For this review, take the finished solid that the model builds, in its own axes (mm). A direction names the side the tool comes from. Round coordinates to 2 decimals unless told otherwise and drop trailing zeros. Write each loop counter-clockwise with the first axis right and the second up, starting at its lowest first coordinate (ties: lowest second). Pieces come first, ordered by that corner, then holes. Notation, with made-up numbers: (-36.5, -24) -> (-13.5, -24) arc R22 cw to (-13.5, -4) -> close; hole circle Ø1 at (56.5, -25.75). An arc over 180 degrees is marked (long way). Answer as CSV lines item,"result". Start each with the question number.
Item 1: For pin 1 Ø1 at (y, z) = (0.5, 21) entering from +X (3 decimals); pin 2 Ø1.6 at (x, y) = (21.5, 1) entering from +Z (3 decimals), all flat-tipped, find the tip position at first contact; note any pin that passes through.
Item 2: Wall thickness on probe 1 along Z at (x, y) = (48.5, 3) (3 decimals); probe 2 along X at (y, z) = (0.25, 67.5) (3 decimals): over which ranges is each line inside the solid? List them lowest first. Write a range as from..to.
Item 3: Take a section at B-B on y = 1.45. Count the separate pieces of the cut face and the enclosed holes in it, then the cut area to 3 significant figures.
Item 4: Machinability: for faces 1 (the flat face through (2, 2, 23)), 2 (the flat face through (86, 2, 71)), 3 (the flat face through (24, 2, 21)), which of the approach directions +Z, -Z, +X, -X, +Y, -Y give a long, thin tool a straight path to every point of the face, cutting with its end or side? Answer none if there is none.
Item 5: Take a section at A-A on x = 69. Give the boundary of the cut face in (y, z) (3 decimals).
Item 6: Mouldability with a two-part tool opening along X and no side actions: class faces 4 (the flat face through (20, 2, 102.35)), 5 (the flat face through (0, 2, 55)), 6 (the flat face through (60, 2, 110)) as +X half, -X half, draft (parallel to the pull), parting line (faces both ways), or undercut.
```python
from build123d import *

# Parameters (mm, degrees)
SKETCH1_W           = 88
SKETCH1_H           = 110
BOSS_EXTRUDE1_DEPTH = 3.175
CUT_EXTRUDE1_REACH  = 5.175
SKETCH2_W           = 8
SKETCH2_H           = 3.175
SKETCH2_W_2         = 3.175
SKETCH2_H_2         = 8
CUT_EXTRUDE2_REACH  = 5.175
SKETCH3_W           = 8
SKETCH3_H           = 3.175
CUT_EXTRUDE3_REACH  = 5.175
SKETCH4_W           = 8
SKETCH4_H           = 3.175


with BuildPart() as part:
    # Sketch1 → Boss-Extrude1 (new body)
    with BuildSketch(Plane(origin=(0, 0, 0), x_dir=(1, 0, 0), z_dir=(0, 1, 0))):
        with Locations((44, -55)):
            Rectangle(SKETCH1_W, SKETCH1_H)
    extrude(amount=BOSS_EXTRUDE1_DEPTH)

    # Sketch2 → Cut-Extrude1 (cut, up to next)
    with BuildSketch(Plane(origin=(0, 3.175, 0), x_dir=(1, 0, 0), z_dir=(0, 1, 0)), mode=Mode.PRIVATE) as cut_extrude1_sk1:
        with Locations((68, -1.5875)):
            Rectangle(SKETCH2_W, SKETCH2_H)
    cut_extrude1_tool1 = extrude(cut_extrude1_sk1.sketch, amount=-CUT_EXTRUDE1_REACH, mode=Mode.PRIVATE) & part.part
    add(cut_extrude1_tool1.solids().sort_by_distance((68, 3.175, 1.5875))[0], mode=Mode.SUBTRACT)
    # Sketch2 → Cut-Extrude1 (cut, up to next)
    with BuildSketch(Plane(origin=(0, 3.175, 0), x_dir=(1, 0, 0), z_dir=(0, 1, 0)), mode=Mode.PRIVATE) as cut_extrude1_sk2:
        with Locations((52, -1.5875)):
            Rectangle(SKETCH2_W, SKETCH2_H)
    cut_extrude1_tool2 = extrude(cut_extrude1_sk2.sketch, amount=-CUT_EXTRUDE1_REACH, mode=Mode.PRIVATE) & part.part
    add(cut_extrude1_tool2.solids().sort_by_distance((52, 3.175, 1.5875))[0], mode=Mode.SUBTRACT)
    # Sketch2 → Cut-Extrude1 (cut, up to next)
    with BuildSketch(Plane(origin=(0, 3.175, 0), x_dir=(1, 0, 0), z_dir=(0, 1, 0)), mode=Mode.PRIVATE) as cut_extrude1_sk3:
        with Locations((20, -1.5875)):
            Rectangle(SKETCH2_W, SKETCH2_H)
    cut_extrude1_tool3 = extrude(cut_extrude1_sk3.sketch, amount=-CUT_EXTRUDE1_REACH, mode=Mode.PRIVATE) & part.part
    add(cut_extrude1_tool3.solids().sort_by_distance((20, 3.175, 1.5875))[0], mode=Mode.SUBTRACT)
    # Sketch2 → Cut-Extrude1 (cut, up to next)
    with BuildSketch(Plane(origin=(0, 3.175, 0), x_dir=(1, 0, 0), z_dir=(0, 1, 0)), mode=Mode.PRIVATE) as cut_extrude1_sk4:
        with Locations((36, -1.5875)):
            Rectangle(SKETCH2_W, SKETCH2_H)
    cut_extrude1_tool4 = extrude(cut_extrude1_sk4.sketch, amount=-CUT_EXTRUDE1_REACH, mode=Mode.PRIVATE) & part.part
    add(cut_extrude1_tool4.solids().sort_by_distance((36, 3.175, 1.5875))[0], mode=Mode.SUBTRACT)
    # Sketch2 → Cut-Extrude1 (cut, up to next)
    with BuildSketch(Plane(origin=(0, 3.175, 0), x_dir=(1, 0, 0), z_dir=(0, 1, 0)), mode=Mode.PRIVATE) as cut_extrude1_sk5:
        with Locations((1.5875, -19)):
            Rectangle(SKETCH2_W_2, SKETCH2_H_2)
    cut_extrude1_tool5 = extrude(cut_extrude1_sk5.sketch, amount=-CUT_EXTRUDE1_REACH, mode=Mode.PRIVATE) & part.part
    add(cut_extrude1_tool5.solids().sort_by_distance((1.5875, 3.175, 19))[0], mode=Mode.SUBTRACT)
    # Sketch2 → Cut-Extrude1 (cut, up to next)
    with BuildSketch(Plane(origin=(0, 3.175, 0), x_dir=(1, 0, 0), z_dir=(0, 1, 0)), mode=Mode.PRIVATE) as cut_extrude1_sk6:
        with Locations((1.5875, -43)):
            Rectangle(SKETCH2_W_2, SKETCH2_H_2)
    cut_extrude1_tool6 = extrude(cut_extrude1_sk6.sketch, amount=-CUT_EXTRUDE1_REACH, mode=Mode.PRIVATE) & part.part
    add(cut_extrude1_tool6.solids().sort_by_distance((1.5875, 3.175, 43))[0], mode=Mode.SUBTRACT)
    # Sketch2 → Cut-Extrude1 (cut, up to next)
    with BuildSketch(Plane(origin=(0, 3.175, 0), x_dir=(1, 0, 0), z_dir=(0, 1, 0)), mode=Mode.PRIVATE) as cut_extrude1_sk7:
        with Locations((1.5875, -91)):
            Rectangle(SKETCH2_W_2, SKETCH2_H_2)
    cut_extrude1_tool7 = extrude(cut_extrude1_sk7.sketch, amount=-CUT_EXTRUDE1_REACH, mode=Mode.PRIVATE) & part.part
    add(cut_extrude1_tool7.solids().sort_by_distance((1.5875, 3.175, 91))[0], mode=Mode.SUBTRACT)
    # Sketch2 → Cut-Extrude1 (cut, up to next)
    with BuildSketch(Plane(origin=(0, 3.175, 0), x_dir=(1, 0, 0), z_dir=(0, 1, 0)), mode=Mode.PRIVATE) as cut_extrude1_sk8:
        with Locations((1.5875, -67)):
            Rectangle(SKETCH2_W_2, SKETCH2_H_2)
    cut_extrude1_tool8 = extrude(cut_extrude1_sk8.sketch, amount=-CUT_EXTRUDE1_REACH, mode=Mode.PRIVATE) & part.part
    add(cut_extrude1_tool8.solids().sort_by_distance((1.5875, 3.175, 67))[0], mode=Mode.SUBTRACT)
    # Sketch2 → Cut-Extrude1 (cut, up to next)
    with BuildSketch(Plane(origin=(0, 3.175, 0), x_dir=(1, 0, 0), z_dir=(0, 1, 0)), mode=Mode.PRIVATE) as cut_extrude1_sk9:
        with Locations((20, -108.4125)):
            Rectangle(SKETCH2_W, SKETCH2_H)
    cut_extrude1_tool9 = extrude(cut_extrude1_sk9.sketch, amount=-CUT_EXTRUDE1_REACH, mode=Mode.PRIVATE) & part.part
    add(cut_extrude1_tool9.solids().sort_by_distance((20, 3.175, 108.4125))[0], mode=Mode.SUBTRACT)
    # Sketch2 → Cut-Extrude1 (cut, up to next)
    with BuildSketch(Plane(origin=(0, 3.175, 0), x_dir=(1, 0, 0), z_dir=(0, 1, 0)), mode=Mode.PRIVATE) as cut_extrude1_sk10:
        with Locations((36, -108.4125)):
            Rectangle(SKETCH2_W, SKETCH2_H)
    cut_extrude1_tool10 = extrude(cut_extrude1_sk10.sketch, amount=-CUT_EXTRUDE1_REACH, mode=Mode.PRIVATE) & part.part
    add(cut_extrude1_tool10.solids().sort_by_distance((36, 3.175, 108.4125))[0], mode=Mode.SUBTRACT)
    # Sketch2 → Cut-Extrude1 (cut, up to next)
    with BuildSketch(Plane(origin=(0, 3.175, 0), x_dir=(1, 0, 0), z_dir=(0, 1, 0)), mode=Mode.PRIVATE) as cut_extrude1_sk11:
        with Locations((68, -108.4125)):
            Rectangle(SKETCH2_W, SKETCH2_H)
    cut_extrude1_tool11 = extrude(cut_extrude1_sk11.sketch, amount=-CUT_EXTRUDE1_REACH, mode=Mode.PRIVATE) & part.part
    add(cut_extrude1_tool11.solids().sort_by_distance((68, 3.175, 108.4125))[0], mode=Mode.SUBTRACT)
    # Sketch2 → Cut-Extrude1 (cut, up to next)
    with BuildSketch(Plane(origin=(0, 3.175, 0), x_dir=(1, 0, 0), z_dir=(0, 1, 0)), mode=Mode.PRIVATE) as cut_extrude1_sk12:
        with Locations((52, -108.4125)):
            Rectangle(SKETCH2_W, SKETCH2_H)
    cut_extrude1_tool12 = extrude(cut_extrude1_sk12.sketch, amount=-CUT_EXTRUDE1_REACH, mode=Mode.PRIVATE) & part.part
    add(cut_extrude1_tool12.solids().sort_by_distance((52, 3.175, 108.4125))[0], mode=Mode.SUBTRACT)
    # Sketch2 → Cut-Extrude1 (cut, up to next)
    with BuildSketch(Plane(origin=(0, 3.175, 0), x_dir=(1, 0, 0), z_dir=(0, 1, 0)), mode=Mode.PRIVATE) as cut_extrude1_sk13:
        with Locations((86.4125, -91)):
            Rectangle(SKETCH2_W_2, SKETCH2_H_2)
    cut_extrude1_tool13 = extrude(cut_extrude1_sk13.sketch, amount=-CUT_EXTRUDE1_REACH, mode=Mode.PRIVATE) & part.part
    add(cut_extrude1_tool13.solids().sort_by_distance((86.4125, 3.175, 91))[0], mode=Mode.SUBTRACT)
    # Sketch2 → Cut-Extrude1 (cut, up to next)
    with BuildSketch(Plane(origin=(0, 3.175, 0), x_dir=(1, 0, 0), z_dir=(0, 1, 0)), mode=Mode.PRIVATE) as cut_extrude1_sk14:
        with Locations((86.4125, -67)):
            Rectangle(SKETCH2_W_2, SKETCH2_H_2)
    cut_extrude1_tool14 = extrude(cut_extrude1_sk14.sketch, amount=-CUT_EXTRUDE1_REACH, mode=Mode.PRIVATE) & part.part
    add(cut_extrude1_tool14.solids().sort_by_distance((86.4125, 3.175, 67))[0], mode=Mode.SUBTRACT)
    # Sketch2 → Cut-Extrude1 (cut, up to next)
    with BuildSketch(Plane(origin=(0, 3.175, 0), x_dir=(1, 0, 0), z_dir=(0, 1, 0)), mode=Mode.PRIVATE) as cut_extrude1_sk15:
        with Locations((86.4125, -19)):
            Rectangle(SKETCH2_W_2, SKETCH2_H_2)
    cut_extrude1_tool15 = extrude(cut_extrude1_sk15.sketch, amount=-CUT_EXTRUDE1_REACH, mode=Mode.PRIVATE) & part.part
    add(cut_extrude1_tool15.solids().sort_by_distance((86.4125, 3.175, 19))[0], mode=Mode.SUBTRACT)
    # Sketch2 → Cut-Extrude1 (cut, up to next)
    with BuildSketch(Plane(origin=(0, 3.175, 0), x_dir=(1, 0, 0), z_dir=(0, 1, 0)), mode=Mode.PRIVATE) as cut_extrude1_sk16:
        with Locations((86.4125, -43)):
            Rectangle(SKETCH2_W_2, SKETCH2_H_2)
    cut_extrude1_tool16 = extrude(cut_extrude1_sk16.sketch, amount=-CUT_EXTRUDE1_REACH, mode=Mode.PRIVATE) & part.part
    add(cut_extrude1_tool16.solids().sort_by_distance((86.4125, 3.175, 43))[0], mode=Mode.SUBTRACT)

    # Sketch3 → Cut-Extrude2 (cut, up to next)
    with BuildSketch(Plane(origin=(0, 3.175, 0), x_dir=(1, 0, 0), z_dir=(0, 1, 0)), mode=Mode.PRIVATE) as cut_extrude2_sk1:
        with Locations((68, -20.7625)):
            Rectangle(SKETCH3_W, SKETCH3_H)
    cut_extrude2_tool1 = extrude(cut_extrude2_sk1.sketch, amount=-CUT_EXTRUDE2_REACH, mode=Mode.PRIVATE) & part.part
    add(cut_extrude2_tool1.solids().sort_by_distance((68, 3.175, 20.7625))[0], mode=Mode.SUBTRACT)
    # Sketch3 → Cut-Extrude2 (cut, up to next)
    with BuildSketch(Plane(origin=(0, 3.175, 0), x_dir=(1, 0, 0), z_dir=(0, 1, 0)), mode=Mode.PRIVATE) as cut_extrude2_sk2:
        with Locations((52, -20.7625)):
            Rectangle(SKETCH3_W, SKETCH3_H)
    cut_extrude2_tool2 = extrude(cut_extrude2_sk2.sketch, amount=-CUT_EXTRUDE2_REACH, mode=Mode.PRIVATE) & part.part
    add(cut_extrude2_tool2.solids().sort_by_distance((52, 3.175, 20.7625))[0], mode=Mode.SUBTRACT)
    # Sketch3 → Cut-Extrude2 (cut, up to next)
    with BuildSketch(Plane(origin=(0, 3.175, 0), x_dir=(1, 0, 0), z_dir=(0, 1, 0)), mode=Mode.PRIVATE) as cut_extrude2_sk3:
        with Locations((20, -20.7625)):
            Rectangle(SKETCH3_W, SKETCH3_H)
    cut_extrude2_tool3 = extrude(cut_extrude2_sk3.sketch, amount=-CUT_EXTRUDE2_REACH, mode=Mode.PRIVATE) & part.part
    add(cut_extrude2_tool3.solids().sort_by_distance((20, 3.175, 20.7625))[0], mode=Mode.SUBTRACT)
    # Sketch3 → Cut-Extrude2 (cut, up to next)
    with BuildSketch(Plane(origin=(0, 3.175, 0), x_dir=(1, 0, 0), z_dir=(0, 1, 0)), mode=Mode.PRIVATE) as cut_extrude2_sk4:
        with Locations((36, -20.7625)):
            Rectangle(SKETCH3_W, SKETCH3_H)
    cut_extrude2_tool4 = extrude(cut_extrude2_sk4.sketch, amount=-CUT_EXTRUDE2_REACH, mode=Mode.PRIVATE) & part.part
    add(cut_extrude2_tool4.solids().sort_by_distance((36, 3.175, 20.7625))[0], mode=Mode.SUBTRACT)

    # Sketch4 → Cut-Extrude3 (cut, up to next)
    with BuildSketch(Plane(origin=(0, 3.175, 0), x_dir=(1, 0, 0), z_dir=(0, 1, 0)), mode=Mode.PRIVATE) as cut_extrude3_sk1:
        with Locations((68, -71.9375)):
            Rectangle(SKETCH4_W, SKETCH4_H)
    cut_extrude3_tool1 = extrude(cut_extrude3_sk1.sketch, amount=-CUT_EXTRUDE3_REACH, mode=Mode.PRIVATE) & part.part
    add(cut_extrude3_tool1.solids().sort_by_distance((68, 3.175, 71.9375))[0], mode=Mode.SUBTRACT)
    # Sketch4 → Cut-Extrude3 (cut, up to next)
    with BuildSketch(Plane(origin=(0, 3.175, 0), x_dir=(1, 0, 0), z_dir=(0, 1, 0)), mode=Mode.PRIVATE) as cut_extrude3_sk2:
        with Locations((52, -71.9375)):
            Rectangle(SKETCH4_W, SKETCH4_H)
    cut_extrude3_tool2 = extrude(cut_extrude3_sk2.sketch, amount=-CUT_EXTRUDE3_REACH, mode=Mode.PRIVATE) & part.part
    add(cut_extrude3_tool2.solids().sort_by_distance((52, 3.175, 71.9375))[0], mode=Mode.SUBTRACT)
    # Sketch4 → Cut-Extrude3 (cut, up to next)
    with BuildSketch(Plane(origin=(0, 3.175, 0), x_dir=(1, 0, 0), z_dir=(0, 1, 0)), mode=Mode.PRIVATE) as cut_extrude3_sk3:
        with Locations((20, -71.9375)):
            Rectangle(SKETCH4_W, SKETCH4_H)
    cut_extrude3_tool3 = extrude(cut_extrude3_sk3.sketch, amount=-CUT_EXTRUDE3_REACH, mode=Mode.PRIVATE) & part.part
    add(cut_extrude3_tool3.solids().sort_by_distance((20, 3.175, 71.9375))[0], mode=Mode.SUBTRACT)
    # Sketch4 → Cut-Extrude3 (cut, up to next)
    with BuildSketch(Plane(origin=(0, 3.175, 0), x_dir=(1, 0, 0), z_dir=(0, 1, 0)), mode=Mode.PRIVATE) as cut_extrude3_sk4:
        with Locations((36, -71.9375)):
            Rectangle(SKETCH4_W, SKETCH4_H)
    cut_extrude3_tool4 = extrude(cut_extrude3_sk4.sketch, amount=-CUT_EXTRUDE3_REACH, mode=Mode.PRIVATE) & part.part
    add(cut_extrude3_tool4.solids().sort_by_distance((36, 3.175, 71.9375))[0], mode=Mode.SUBTRACT)
    # Sketch4 → Cut-Extrude3 (cut, up to next)
    with BuildSketch(Plane(origin=(0, 3.175, 0), x_dir=(1, 0, 0), z_dir=(0, 1, 0)), mode=Mode.PRIVATE) as cut_extrude3_sk5:
        with Locations((68, -100.7625)):
            Rectangle(SKETCH4_W, SKETCH4_H)
    cut_extrude3_tool5 = extrude(cut_extrude3_sk5.sketch, amount=-CUT_EXTRUDE3_REACH, mode=Mode.PRIVATE) & part.part
    add(cut_extrude3_tool5.solids().sort_by_distance((68, 3.175, 100.7625))[0], mode=Mode.SUBTRACT)
    # Sketch4 → Cut-Extrude3 (cut, up to next)
    with BuildSketch(Plane(origin=(0, 3.175, 0), x_dir=(1, 0, 0), z_dir=(0, 1, 0)), mode=Mode.PRIVATE) as cut_extrude3_sk6:
        with Locations((52, -100.7625)):
            Rectangle(SKETCH4_W, SKETCH4_H)
    cut_extrude3_tool6 = extrude(cut_extrude3_sk6.sketch, amount=-CUT_EXTRUDE3_REACH, mode=Mode.PRIVATE) & part.part
    add(cut_extrude3_tool6.solids().sort_by_distance((52, 3.175, 100.7625))[0], mode=Mode.SUBTRACT)
    # Sketch4 → Cut-Extrude3 (cut, up to next)
    with BuildSketch(Plane(origin=(0, 3.175, 0), x_dir=(1, 0, 0), z_dir=(0, 1, 0)), mode=Mode.PRIVATE) as cut_extrude3_sk7:
        with Locations((20, -100.7625)):
            Rectangle(SKETCH4_W, SKETCH4_H)
    cut_extrude3_tool7 = extrude(cut_extrude3_sk7.sketch, amount=-CUT_EXTRUDE3_REACH, mode=Mode.PRIVATE) & part.part
    add(cut_extrude3_tool7.solids().sort_by_distance((20, 3.175, 100.7625))[0], mode=Mode.SUBTRACT)
    # Sketch4 → Cut-Extrude3 (cut, up to next)
    with BuildSketch(Plane(origin=(0, 3.175, 0), x_dir=(1, 0, 0), z_dir=(0, 1, 0)), mode=Mode.PRIVATE) as cut_extrude3_sk8:
        with Locations((36, -100.7625)):
            Rectangle(SKETCH4_W, SKETCH4_H)
    cut_extrude3_tool8 = extrude(cut_extrude3_sk8.sketch, amount=-CUT_EXTRUDE3_REACH, mode=Mode.PRIVATE) & part.part
    add(cut_extrude3_tool8.solids().sort_by_distance((36, 3.175, 100.7625))[0], mode=Mode.SUBTRACT)


solid = part.part
```
Output values:
1,pin 1,"stops at x = 84.825"
1,pin 2,"stops at z = 106.825"
2,probe 1,"z = 3.175..19.175, 22.35..70.35, 73.525..99.175, 102.35..106.825"
2,probe 2,"x = 3.175..84.825"
3,separate pieces,"1"
3,enclosed holes,"12"
3,area,"8,970 mm^2"
4,face 1,"-X, +Y, -Y"
4,face 2,"+X, +Y, -Y"
4,face 3,"+Y, -Y"
5,outline,"(0, 3.175) -> (3.175, 3.175) -> (3.175, 19.175) -> (0, 19.175) -> close; (0, 22.35) -> (3.175, 22.35) -> (3.175, 70.35) -> (0, 70.35) -> close; (0, 73.525) -> (3.175, 73.525) -> (3.175, 99.175) -> (0, 99.175) -> close; (0, 102.35) -> (3.175, 102.35) -> (3.175, 106.825) -> (0, 106.825) -> close"
6,face 4,"undercut"
6,face 5,"-X half"
6,face 6,"draft"
